Build history of the part. All positions in model axes, mm. A direction names the side the tool comes from. Round coordinates to 2 decimals unless told otherwise and drop trailing zeros. Write each loop counter-clockwise with the first axis right and the second up, starting at its lowest first coordinate (ties: lowest second). Pieces come first, ordered by that corner, then holes. Notation, with made-up numbers: (-36, -30.5) -> (13, -30.5) arc R12 ccw to (13, -24.5) -> close; hole circle Ø11 at (86.5, -10.5). An arc over 180 degrees is marked (long way). Answer in a Markdown table with one row per item.
```python
from build123d import *

# Parameters (mm, degrees)
BOSS_EXTRUDE2_DEPTH                          = 6.5
SKETCH2_R                                    = 23
SKETCH2_R_2                                  = 10
BOSS_EXTRUDE3_DEPTH                          = 9.5
BOSS_EXTRUDE4_DEPTH                          = 24
CHAMFER2_SIZE                                = 1
CSK_FOR_M3_COUNTERSUNK_RAISED_HEAD_S_2_COUNT = 2
CSK_FOR_M3_COUNTERSUNK_RAISED_HEAD_S_2_PITCH = 25
CHAMFER2_OF_MIRROR4_SIZE                     = 1
SKETCH4_R                                    = 20
CUT_EXTRUDE1_DEPTH                           = 126.420293414
CUT_EXTRUDE2_DEPTH                           = 9
CUT_EXTRUDE3_REACH                           = 125.366
CUT_EXTRUDE3_END_RADIUS                      = 20
SKETCH6_5_R                                  = 5
CHAMFER3_SIZE                                = 1


with BuildPart() as part:
    # Sketch1 → Boss-Extrude2 (new, symmetric)
    with BuildSketch(Plane(origin=(0, 0, 0), x_dir=(1, 0, 0), z_dir=(0, 1, 0))):
        with BuildLine():
            ThreePointArc((-23, 0), (0, -23), (23, 0))
            Line((23, 0), (34, -75))
            Line((34, -75), (-34, -75))
            Line((-34, -75), (-23, 0))
        make_face()
    boss_extrude2 = extrude(amount=BOSS_EXTRUDE2_DEPTH, both=True)

    # Sketch2 → Boss-Extrude3 (add, symmetric)
    with BuildSketch(Plane(origin=(0, 0, 0), x_dir=(1, 0, 0), z_dir=(0, 1, 0))):
        with Locations(Location((0, 0, 0), (0, 0, 270))):
            Circle(SKETCH2_R)
        with Locations(Location((0, 0, 0), (0, 0, 270))):
            Circle(SKETCH2_R_2, mode=Mode.SUBTRACT)
    boss_extrude3 = extrude(amount=BOSS_EXTRUDE3_DEPTH, both=True)

    # Sketch3 → Boss-Extrude4 (add)
    with BuildSketch(Plane(origin=(0, 6.5, 0), x_dir=(1, 0, 0), z_dir=(0, 1, 0))):
        Polygon((-29.6, -45), (29.6, -45), (34, -75), (-34, -75), align=None)
    boss_extrude4 = extrude(amount=BOSS_EXTRUDE4_DEPTH)

    # Chamfer2
    chamfer2_edges = [part.edges().sort_by_distance(p)[0] for p in [
        (0, -9.5, -10),
    ]]
    chamfer(chamfer2_edges, length=CHAMFER2_SIZE)

    # Sketch12 → CSK for M3 Countersunk Raised Head Screw2 (revolve, cut)
    with BuildSketch(Plane(origin=(10, -9.5, -12.5), x_dir=(0, 0, -1), z_dir=(1, 0, 0))):
        Polygon((0, 0), (0, 12), (1.7, 10.978536948), (1.7, 1.45), (3.15, 0), align=None)
    csk_for_m3_countersunk_raised_head_screw = revolve(axis=Axis((10, -15.85, -12.5), (0, 1, 0)), mode=Mode.SUBTRACT)

    # CSK for M3 Countersunk Raised Head S 2: CSK for M3 Countersunk Raised Head Screw2 ×2
    with Locations(*[(0, 0, i * CSK_FOR_M3_COUNTERSUNK_RAISED_HEAD_S_2_PITCH) for i in range(1, CSK_FOR_M3_COUNTERSUNK_RAISED_HEAD_S_2_COUNT)]):
        add(csk_for_m3_countersunk_raised_head_screw, mode=Mode.SUBTRACT)

    # Mirror4: Boss-Extrude2, Boss-Extrude3, Boss-Extrude4, CSK for M3 Countersunk Raised Head Screw2 across plane
    add(boss_extrude2.mirror(Plane.ZX.offset(30.5)))
    add(boss_extrude3.mirror(Plane.ZX.offset(30.5)))
    add(boss_extrude4.mirror(Plane.ZX.offset(30.5)))
    add(csk_for_m3_countersunk_raised_head_screw.mirror(Plane.ZX.offset(30.5)), mode=Mode.SUBTRACT)

    # Mirror4 copy 1 sketch → Mirror4 copy 1 (revolve, cut)
    with BuildSketch(Plane(origin=(10, 70.5, 12.5), x_dir=(0, 0, -1), z_dir=(1, 0, 0))):
        Polygon((0, 0), (0, -12), (1.7, -10.978536948), (1.7, -1.45), (3.15, 0), align=None)
    revolve(axis=Axis((10, 76.85, 12.5), (0, 1, 0)), mode=Mode.SUBTRACT)

    # Chamfer2 of Mirror4
    chamfer2_of_mirror4_edges = [part.edges().sort_by_distance(p)[0] for p in [
        (0, 70.5, -10),
    ]]
    chamfer(chamfer2_of_mirror4_edges, length=CHAMFER2_OF_MIRROR4_SIZE)

    # Sketch4 → Cut-Extrude1 (cut, through all)
    with BuildSketch(Plane.XY.offset(75)):
        with Locations((0, 30.5)):
            Circle(SKETCH4_R)
    extrude(amount=-CUT_EXTRUDE1_DEPTH, mode=Mode.SUBTRACT)

    # Sketch6 → Cut-Extrude2 (cut)
    with BuildSketch(Plane(origin=(34, 0, 0), x_dir=(0, 0, -1), z_dir=(1, 0, 0))):
        with BuildLine():
            Line((-60, 43), (-45, 43))
            Line((-45, 43), (-45, 18))
            Line((-45, 18), (-60, 18))
            ThreePointArc((-60, 18), (-72.5, 30.5), (-60, 43))
        make_face()
    extrude(amount=-CUT_EXTRUDE2_DEPTH, mode=Mode.SUBTRACT)

    # Cut-Extrude3: up to this cylinder (the profile starts outside it)
    cut_extrude3_end = Plane(origin=(0, 30.5, 60), z_dir=(0, 0, 1)) * Cylinder(CUT_EXTRUDE3_END_RADIUS, 291.732, mode=Mode.PRIVATE)
    # Sketch6<5> → Cut-Extrude3 (cut, up to the surface)
    with BuildSketch(Plane(origin=(34, 0, 0), x_dir=(0, 0, -1), z_dir=(1, 0, 0)), mode=Mode.PRIVATE) as cut_extrude3_sk1:
        with Locations((-60, 30.5)):
            Circle(SKETCH6_5_R)
    cut_extrude3_tool1 = extrude(cut_extrude3_sk1.sketch, amount=-CUT_EXTRUDE3_REACH, mode=Mode.PRIVATE) - cut_extrude3_end
    add(cut_extrude3_tool1.solids().sort_by_distance((34, 30.5, 60))[0], mode=Mode.SUBTRACT)

    # Chamfer3
    chamfer3_edges = [part.edges().sort_by_distance(p)[0] for p in [
        (-20, 30.5, 75),
    ]]
    chamfer(chamfer3_edges, length=CHAMFER3_SIZE)


solid = part.part
```
Q1. Saw through at C-C on z = 19. Write the cut outline in (x, y).
A:
| item | result |
|---|---|
| outline | (-25.79, -6.5) -> (-12.96, -6.5) -> (-12.96, -9.5) -> (12.96, -9.5) -> (12.96, -6.5) -> (25.79, -6.5) -> (25.79, 6.5) -> (12.96, 6.5) -> (12.96, 9.5) -> (-12.96, 9.5) -> (-12.96, 6.5) -> (-25.79, 6.5) -> close; (-25.79, 54.5) -> (-12.96, 54.5) -> (-12.96, 51.5) -> (12.96, 51.5) -> (12.96, 54.5) -> (25.79, 54.5) -> (25.79, 67.5) -> (12.96, 67.5) -> (12.96, 70.5) -> (-12.96, 70.5) -> (-12.96, 67.5) -> (-25.79, 67.5) -> close |
Q2. Saw through at B-B on x = 0. State how many separate pieces and enclosed holes the cut face has, plus the area to 3 significant figures.
A:
| item | result |
|---|---|
| separate pieces | 4 |
| enclosed holes | 0 |
| area | 2,580 mm² |
Q3. Two-plate mould, pull along Y, no slides. Class faces 5 (the flat face through (-5, 9.5, 10)), 6 (the flat face through (0, 67.5, 45)), 7 (the cylindrical face through (-2.6, 50.33, 59.7)), 8 (the flat face through (-29.8, 31.02, 46.36)): released by +Y, released by -Y, zero draft, split by the parting line, or undercut.
A:
| item | result |
|---|---|
| face 5 | undercut |
| face 6 | released by +Y |
| face 7 | undercut |
| face 8 | zero draft |
Q4. Drop flat-ended pins along their axis: P1, Ø12, axis at x = 26.5, y = -0.5, coming from the -Z side; P2, Ø5, axis at y = 58.5, z = 60, coming from the -X side; P3, Ø8, axis at y = 24.5, z = 55, coming from the +X side. Give the stop position or say it passes through.
A:
| item | result |
|---|---|
| P1 | z = -10.43 |
| P2 | x = -32.17 |
| P3 | x = 25 |
Q5. Which spindle directions (+Z, -Z, +X, -X, +Y, -Y) get a long thin tool onto all of the face, cutting with end or side? Do faces 1 (the flat face through (-5, 51.5, 10)), 2 (the flat face through (25, 33.5, 55.5)), 3 (the cylindrical face through (11.5, -3.4, -13.3)), 4 (the cylindrical face through (22.222, 35.457, 60.651)). Say none if no direction does.
A:
| item | result |
|---|---|
| face 1 | -Z, +X, -X |
| face 2 | -Z, +X |
| face 3 | -Y |
| face 4 | +X |
Q6. Wall check: line 1 (Y direction, x = -2, z = 13); line 2 (Y direction, x = 0, z = 23.5); line 3 (Z direction, x = -22, y = 22.5). Give the ranges that are in metal, low to high. Write a range as [from, to].
A:
| item | result |
|---|---|
| line 1 | [-9.5, 9.5], [51.5, 70.5] |
| line 2 | [-6.5, 6.5], [54.5, 67.5] |
| line 3 | [45, 75] |
Q7. Saw through at A-A on y = 62.5. Write the cut outline in (x, z), plus the area to 3 significant figures.
A:
| item | result |
|---|---|
| outline | (-34, 75) -> (-23, 0) arc R23 ccw to (23, 0) -> (34, 75) -> close; hole circle Ø20 at (0, 0); hole circle Ø3.4 at (10, -12.5); hole circle Ø3.4 at (10, 12.5) |
| area | 4,770 mm² |
